Input: part model. Units: mm. Frame: model coordinates. Give positions to 0.01 mm unless a question says otherwise; leave off trailing zeros. Loops run counter-clockwise (first coordinate to the right, second up) from the corner with the lowest first, then second, coordinate; pieces in that order, holes last. Notation, with made-up numbers: M -26.75,41.25 L 11.25,41.25 A10 ccw 11.25,46.25 Z; hole C -4,75.5 d8. An arc over 180 degrees is marked long. Use CSV: the item, a comma, the result in double quotes. Start each with the question number.
Q1. Material intervals for line 1 along X through (y, z) = (17, 20); line 2 along Z through (x, y) = (16.5, 11.5); line 3 along Z through (x, y) = (12.5, 30), sorted ascending.
Q2. Section B-B, the plane z = 23. Output: boundary loops of the cut face in (x, y), plus the area to 3 significant figures.
Q3. Pin query (flat end, axial travel): pin 1 (1.5 mm diameter, centred on x = 25, y = 10.5, fed in from +Z); pin 2 (1 mm diameter, centred on x = 14.5, z = 62, fed in from -Y); pin 3 (3 mm diameter, centred on x = 8.5, y = 4, fed in from +Z). Return the tip coordinate at first contact, or that it passes through.
Q4. Section C-C, the plane y = 24. Output: boundary loops of the cut face in (x, z).
Q5. Section A-A, the plane y = 7. Output: boundary loops of the cut face in (x, z), plus the area to 3 significant figures.
Q6. Section D-D, the plane x = 11.5. Output: boundary loops of the cut face in (y, z), plus the area to 3 significant figures.
Q7. Pull-direction query (Z, two-part tool) for faces 1 (the cylindrical face through (15, 16, 63)), 2 (the flat face through (15, 40, 66)), 3 (the flat face through (27, 20, 2)); classes: released by +Z, released by -Z, zero draft, split by the parting line, or undercut.
from build123d import *

# Parameters (mm, degrees)
SALIENTE_EXTRUIR1_DEPTH    = 30
CORTAR_EXTRUIR1_DEPTH      = 54
CORTAR_EXTRUIR1_DEPTH_BACK = 94
CROQUIS2_R                 = 9.5
CORTAR_EXTRUIR2_DEPTH      = 94
CORTAR_EXTRUIR2_DEPTH_BACK = 94
CROQUIS3_R                 = 15
CROQUIS3_R_2               = 16
CHAFL_N1_SIZE              = 5


with BuildPart() as part:
    # Croquis1 → Saliente-Extruir1 (new body)
    with BuildSketch(Plane(origin=(0, 0, 0), x_dir=(0, 0, -1), z_dir=(1, 0, 0))):
        Polygon((-100, 0), (-82, 40), (0, 40), (0, 0), align=None)
    extrude(amount=SALIENTE_EXTRUIR1_DEPTH)

    # Croquis2 → Cortar-Extruir1 (cut, two sides: drawn at the far end of the back side and taken through both)
    with BuildSketch(Plane(origin=(0, 40, 0), x_dir=(1, 0, 0), z_dir=(0, 1, 0)).offset(-CORTAR_EXTRUIR1_DEPTH_BACK)):
        with Locations((15, -100)):
            Circle(CROQUIS2_R)
        with Locations(Location((15, -20, 0), (0, 0, 90))):
            Circle(CROQUIS2_R)
    extrude(amount=CORTAR_EXTRUIR1_DEPTH + CORTAR_EXTRUIR1_DEPTH_BACK, mode=Mode.SUBTRACT)

    # Croquis3 → Cortar-Extruir2 (cut, two sides: drawn at the far end of the back side and taken through both)
    with BuildSketch(Plane(origin=(30, 0, 0), x_dir=(0, 0, -1), z_dir=(1, 0, 0)).offset(-CORTAR_EXTRUIR2_DEPTH_BACK)):
        with Locations((-35, 40)):
            Circle(CROQUIS3_R)
        with Locations((-63, 0)):
            Circle(CROQUIS3_R_2)
    extrude(amount=CORTAR_EXTRUIR2_DEPTH + CORTAR_EXTRUIR2_DEPTH_BACK, mode=Mode.SUBTRACT)

    # Chafl_n1
    chafl_n1_edges = [part.edges().sort_by_distance(p)[0] for p in [
        (30, 20, 0),
        (0, 20, 0),
    ]]
    chamfer(chafl_n1_edges, length=CHAFL_N1_SIZE)


solid = part.part
A:
1,line 1,"0 to 5.5, 24.5 to 30"
1,line 2,"0 to 10.62, 29.38 to 51.88, 74.12 to 90.62"
1,line 3,"0 to 10.83, 46.18 to 86.5"
2,outline,"M 0,0 L 5.99,0 L 5.99,31 L 0,31 Z; M 24.01,0 L 30,0 L 30,31 L 24.01,31 Z"
2,area,"371 mm^2"
3,pin 1,"z = 95.61"
3,pin 2,"y = 15.93"
3,pin 3,"z = 94.88"
4,outline,"M 0,5 L 5,0 L 25,0 L 30,5 L 30,89.2 L 0,89.2 Z; hole C 15,20 d19"
5,outline,"M 0,5 L 5,0 L 25,0 L 30,5 L 30,48.61 L 0,48.61 Z; M 0,77.39 L 30,77.39 L 30,96.85 L 23.96,96.85 A9.5 cw 6.04,96.85 L 0,96.85 Z; hole C 15,20 d19"
5,area,"1,650 mm^2"
6,outline,"M 0,0 L 40,0 L 40,11.17 L 0,11.17 Z; M 0,28.83 L 26.33,28.83 A15 cw 40,50 L 40,82 L 19.63,91.17 L 0,91.17 L 0,79 A16 cw 0,47 Z"
6,area,"2,180 mm^2"
7,face 1,"undercut"
7,face 2,"zero draft"
7,face 3,"released by -Z"
